Read the model definition and answer for the solid it produces. Units are mm, in the model's axes. A direction names the side the tool comes from. Round coordinates to 2 decimals unless told otherwise and drop trailing zeros. Loops run counter-clockwise (first coordinate to the right, second up) from the corner with the lowest first, then second, coordinate; pieces in that order, holes last. Notation, with made-up numbers: M 83,72 L 93,72 A21 ccw 93,83 Z; hole C 45,32 d10. An arc over 180 degrees is marked long. Write each question's results on one line, items separated by ' | '.
from build123d import *

# Parameters (mm, degrees)
SKETCH_1_W           = 25.4
SKETCH_1_H           = 3
EXTRUDE_1_DEPTH      = 8.4
EXTRUDE_1_2_DEPTH    = 8.4
EXTRUDE_2_DEPTH      = 3
EXTRUDE_2_DEPTH_BACK = 3
FILLET_1_R           = 2
SKETCH_3_R           = 2.1
CUT_EXTRUDE_1_DEPTH  = 6


with BuildPart() as part:
    # Sketch 1 → Extrude 1 (new body)
    with BuildSketch(Plane(origin=(0, 0, 0), x_dir=(1, 0, 0), z_dir=(0, 1, 0))):
        with Locations((-63.521674557, 78.184540652)):
            Rectangle(SKETCH_1_W, SKETCH_1_H)
    extrude(amount=EXTRUDE_1_DEPTH)



with BuildPart() as body_2:
    # Sketch 1 → Extrude 1 2 (new body)
    with BuildSketch(Plane(origin=(0, 0, 0), x_dir=(1, 0, 0), z_dir=(0, 1, 0))):
        with Locations((-63.521674557, 43.184540652)):
            Rectangle(SKETCH_1_W, SKETCH_1_H)
    extrude(amount=EXTRUDE_1_2_DEPTH)


with BuildPart() as part_1:
    add(part.part)

    add(body_2.part)  # Extrude 2 merges body 2
    # Sketch 2 → Extrude 2 (add, two sides: drawn at the far end of the back side and taken through both)
    with BuildSketch(Plane(origin=(0, 8.4, 0), x_dir=(1, 0, 0), z_dir=(0, 1, 0)).offset(-EXTRUDE_2_DEPTH_BACK)):
        Polygon((-40.821674557, 55.684540652), (-40.821674557, 41.684540652), (-50.821674557, 41.684540652), (-50.821674557, 79.684540652), (-40.821674557, 79.684540652), (-40.821674557, 65.684540652), (-30.821674557, 65.684540652), (-30.821674557, 55.684540652), align=None)
    extrude(amount=EXTRUDE_2_DEPTH + EXTRUDE_2_DEPTH_BACK)

    # Fillet 1
    fillet_1_edges = [part_1.edges().sort_by_distance(p)[0] for p in [
        (-50.821674557, 8.4, -78.184540652),
        (-50.821674557, 5.4, -78.184540652),
        (-40.821674557, 8.4, -79.684540652),
        (-40.821674557, 8.4, -65.684540652),
        (-30.821674557, 8.4, -65.684540652),
        (-30.821674557, 8.4, -55.684540652),
        (-40.821674557, 8.4, -55.684540652),
        (-40.821674557, 8.4, -41.684540652),
        (-50.821674557, 5.4, -43.184540652),
        (-50.821674557, 8.4, -43.184540652),
    ]]
    fillet(fillet_1_edges, radius=FILLET_1_R)

    # Sketch 3 → Cut-Extrude 1 (cut)
    with BuildSketch(Plane(origin=(0, 11.4, 0), x_dir=(1, 0, 0), z_dir=(0, 1, 0))):
        with Locations(Location((-45.821674557, 60.684540652, 0), (0, 0, 270))):
            Circle(SKETCH_3_R)
        with Locations(Location((-35.821674557, 60.684540652, 0), (0, 0, 270))):
            Circle(SKETCH_3_R)
    extrude(amount=-CUT_EXTRUDE_1_DEPTH, mode=Mode.SUBTRACT)


solid = part_1.part
Item 1: Flat-ended cylindrical pins translate along their axes: pin 1 (6.5 mm diameter, centred on y = 9, z = -47.5, fed in from +X); pin 2 (6 mm diameter, centred on y = 10, z = -71.5, fed in from -X); pin 3 (6.5 mm diameter, centred on x = -36, y = 7, fed in from +Z). Find the tip coordinate at first contact, or state that the pin passes through.
Outcome:
pin 1: stops at x = -40.82 | pin 2: stops at x = -50.82 | pin 3: stops at z = -55.64
Item 2: Straight lines are drawn through the part: line 1 (Z direction, x = -54, y = 7.25); line 2 (Y direction, x = -49, z = -58); line 3 (X direction, y = 10.75, z = -72.5). For each, find the intervals that lie inside material, in ascending order.
Outcome:
line 1: z = -79.68 to -76.68, -44.68 to -41.68 | line 2: y = 5.4 to 11.4 | line 3: x = -50.82 to -40.82
Item 3: The part is cut by section C-C (y = 2.75). Determine the outline of the cut face in (x, z).
Outcome:
outline: M -76.22,-79.68 L -50.82,-79.68 L -50.82,-76.68 L -76.22,-76.68 Z; M -76.22,-44.68 L -50.82,-44.68 L -50.82,-41.68 L -76.22,-41.68 Z
Item 4: The part is cut by section D-D (y = 9.25). Determine the outline of the cut face in (x, z).
Outcome:
outline: M -51.19,-79.68 L -42.82,-79.68 A2 ccw -40.82,-77.68 L -40.82,-67.68 A2 cw -38.82,-65.68 L -32.82,-65.68 A2 ccw -30.82,-63.68 L -30.82,-57.68 A2 ccw -32.82,-55.68 L -38.82,-55.68 A2 cw -40.82,-53.68 L -40.82,-43.68 A2 ccw -42.82,-41.68 L -51.19,-41.68 L -51.19,-44.68 L -50.82,-44.68 L -50.82,-76.68 L -51.19,-76.68 Z; hole C -45.82,-60.68 d4.2; hole C -35.82,-60.68 d4.2
Item 5: The part is cut by section A-A (x = -62). Determine the outline of the cut face in (y, z).
Outcome:
outline: M 0,-79.68 L 8.4,-79.68 L 8.4,-76.68 L 0,-76.68 Z; M 0,-44.68 L 8.4,-44.68 L 8.4,-41.68 L 0,-41.68 Z
Item 6: The mould has two halves that part along X. Classify faces 1 (the face through (-50.22, 4.83, -78.21)), 2 (the face through (-33.74, 8.44, -60.96)), 3 (the face through (-63, 4, -44.685)): pulls with the +X half, pulls with the -X half, needs draft (parallel to the pull), parting line crosses it, or undercut.
Outcome:
face 1: pulls with the +X half | face 2: undercut | face 3: needs draft
Item 7: For faces 4 (the face through (-40.822, 8, -49)), 5 (the face through (-40.822, 8, -73)), 6 (the face through (-65, 8.4, -78)), determine the directions among +Z, -Z, +X, -X, +Y, -Y from which every point of the face is accessible in a straight line to the end or side of a thin tool.
Outcome:
face 4: +Z, +X, +Y, -Y | face 5: -Z, +X, +Y, -Y | face 6: +Z, -Z, -X, +Y
Item 8: The part is cut by section B-B (z = -60). Determine the outline of the cut face in (x, y).
Outcome:
outline: M -50.82,5.4 L -47.81,5.4 L -47.81,11.4 L -50.82,11.4 Z; M -43.84,5.4 L -37.81,5.4 L -37.81,11.4 L -43.84,11.4 Z; M -33.84,5.4 L -30.82,5.4 L -30.82,11.4 L -33.84,11.4 Z
